For this review, take the finished solid that the model builds, in its own axes (mm). Face numbers are marked on the shaded views. Round coordinates to 2 decimals unless told otherwise and drop trailing zeros. Loops run counter-clockwise (first coordinate to the right, second up) from the corner with the lowest first, then second, coordinate; pieces in that order, holes last. Notation, with made-up numbers: (-0.5, 26.5) -> (14.5, 26.5) arc R29 cw to (14.5, 50.5) -> close; hole circle Ø2 at (82, 39.25). An arc over 180 degrees is marked (long way). Use one line per item in the form item = value. Start each with the question number.
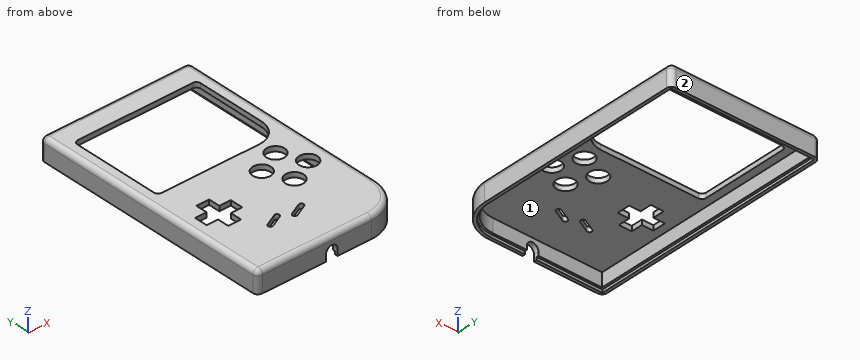
from build123d import *

# Parameters (mm, degrees)
SKETCH1_W               = 90
SKETCH1_H               = 147.5
BOSS_EXTRUDE1_DEPTH     = 13
ROUNDED_BOTTOM_CORNER_R = 21
ROUND_EDGES_R           = 3
SHELL2_DEPTH            = 10
CUT_EXTRUDE1_DEPTH      = 88.367399526
CUT_EXTRUDE2_DEPTH      = 1.75
CUT_EXTRUDE3_REACH      = 156.759
SKETCH6_R               = 5.5
CUT_EXTRUDE4_DEPTH      = 88.367399526
SKETCH7_W               = 7.75
SKETCH7_H               = 21.6
SKETCH7_W_2             = 21.6
SKETCH7_H_2             = 7.75
CUT_EXTRUDE5_DEPTH      = 88.367399526
CUT_EXTRUDE6_DEPTH      = 88.367399526


# Read off the part's stored shape, not the designer's step: Shell2
with BuildPart() as part:
    # Sketch1 → Boss-Extrude1 (new body)
    with BuildSketch(Plane.XY):
        Rectangle(SKETCH1_W, SKETCH1_H)
    extrude(amount=BOSS_EXTRUDE1_DEPTH)

    # Rounded Bottom Corner
    rounded_bottom_corner_edges = [part.edges().sort_by_distance(p)[0] for p in [
        (45, -73.75, 6.5),
    ]]
    fillet(rounded_bottom_corner_edges, radius=ROUNDED_BOTTOM_CORNER_R)

    # Round Edges
    round_edges_edges = [part.edges().sort_by_distance(p)[0] for p in [
        (-45, 0, 13),
        (-10.5, -73.75, 13),
        (45, 10.5, 13),
        (38.849242405, -67.599242405, 13),
        (0, 73.75, 13),
        (-45, -73.75, 6.5),
        (-45, 73.75, 6.5),
        (45, 73.75, 6.5),
    ]]
    fillet(round_edges_edges, radius=ROUND_EDGES_R)

    # Shell2 outline → Shell2 (cut)
    with BuildSketch(Plane.XY):
        with BuildLine():
            Line((42, -52.75), (42, 70.75))
            Line((42, 70.75), (-42, 70.75))
            Line((-42, 70.75), (-42, -70.75))
            Line((-42, -70.75), (24, -70.75))
            ThreePointArc((24, -70.75), (36.727922061, -65.477922061), (42, -52.75))
        make_face()
    extrude(amount=SHELL2_DEPTH, mode=Mode.SUBTRACT)

    # Sketch2 → Cut-Extrude1 (cut, through all)
    with BuildSketch(Plane.XY.offset(13)):
        with BuildLine():
            Line((-34.75, 59.75), (34.75, 59.75))
            ThreePointArc((34.75, 59.75), (36.517766953, 59.017766953), (37.25, 57.25))
            Line((37.25, 57.25), (37.25, 15.75))
            ThreePointArc((37.25, 15.75), (33.442388155, 6.557611845), (24.25, 2.75))
            Line((24.25, 2.75), (-34.75, 2.75))
            ThreePointArc((-34.75, 2.75), (-36.517766953, 3.482233047), (-37.25, 5.25))
            Line((-37.25, 5.25), (-37.25, 57.25))
            ThreePointArc((-37.25, 57.25), (-36.517766953, 59.017766953), (-34.75, 59.75))
        make_face()
    extrude(amount=-CUT_EXTRUDE1_DEPTH, mode=Mode.SUBTRACT)

    # Sketch3 → Cut-Extrude2 (cut)
    with BuildSketch(Plane(origin=(0, 0, 0), x_dir=(-1, 0, 0), z_dir=(0, 0, -1))):
        with BuildLine():
            Line((-43.25, -52.75), (-43.25, 72))
            Line((-43.25, 72), (43.25, 72))
            Line((43.25, 72), (43.25, -72))
            Line((43.25, -72), (-24, -72))
            ThreePointArc((-24, -72), (-37.611805538, -66.361805538), (-43.25, -52.75))
        make_face()
        with BuildLine():
            Line((-42, -52.75), (-42, 70.75))
            Line((-42, 70.75), (42, 70.75))
            Line((42, 70.75), (42, -70.75))
            Line((42, -70.75), (-24, -70.75))
            ThreePointArc((-24, -70.75), (-36.727922061, -65.477922061), (-42, -52.75))
        make_face(mode=Mode.SUBTRACT)
    extrude(amount=-CUT_EXTRUDE2_DEPTH, mode=Mode.SUBTRACT)

    # Sketch4 → Cut-Extrude3 (cut, up to next)
    with BuildSketch(Plane.XZ.offset(73.75), mode=Mode.PRIVATE) as cut_extrude3_sk1:
        with BuildLine():
            Line((-3.5, 0), (3.5, 0))
            Line((3.5, 0), (3.5, 4))
            ThreePointArc((3.5, 4), (0, 7.5), (-3.5, 4))
            Line((-3.5, 4), (-3.5, 0))
        make_face()
    cut_extrude3_tool1 = extrude(cut_extrude3_sk1.sketch, amount=-CUT_EXTRUDE3_REACH, mode=Mode.PRIVATE) & part.part
    add(cut_extrude3_tool1.solids().sort_by_distance((0, -73.75, 3.419658))[0], mode=Mode.SUBTRACT)

    # Sketch6 → Cut-Extrude4 (cut, through all)
    with BuildSketch(Plane.XY.offset(13)):
        with Locations((32, -21.75)):
            Circle(SKETCH6_R)
        with Locations((17.546893068, -28.66)):
            Circle(SKETCH6_R)
        with Locations((25.098626717, -7.314936896)):
            Circle(SKETCH6_R)
        with Locations((10.645519784, -14.224936896)):
            Circle(SKETCH6_R)
    extrude(amount=-CUT_EXTRUDE4_DEPTH, mode=Mode.SUBTRACT)

    # Sketch7 → Cut-Extrude5 (cut, through all)
    with BuildSketch(Plane.XY.offset(13)):
        with Locations((-26.15, -26.31)):
            Rectangle(SKETCH7_W, SKETCH7_H)
        with Locations((-26.15, -26.31)):
            Rectangle(SKETCH7_W_2, SKETCH7_H_2)
    extrude(amount=-CUT_EXTRUDE5_DEPTH, mode=Mode.SUBTRACT)

    # Sketch8 → Cut-Extrude6 (cut, through all)
    with BuildSketch(Plane.XY.offset(13)):
        with BuildLine():
            Line((-2.01359375, -48.949501032), (5.145672972, -45.379501032))
            ThreePointArc((5.145672972, -45.379501032), (6.98976569, -45.99640625), (6.372860472, -47.840498968))
            Line((6.372860472, -47.840498968), (-0.78640625, -51.410498968))
            ThreePointArc((-0.78640625, -51.410498968), (-2.630498968, -50.79359375), (-2.01359375, -48.949501032))
        make_face()
        with BuildLine():
            Line((-15.98359375, -48.099501032), (-8.824327028, -44.529501032))
            ThreePointArc((-8.824327028, -44.529501032), (-6.98023431, -45.14640625), (-7.597139528, -46.990498968))
            Line((-7.597139528, -46.990498968), (-14.75640625, -50.560498968))
            ThreePointArc((-14.75640625, -50.560498968), (-16.600498968, -49.94359375), (-15.98359375, -48.099501032))
        make_face()
    extrude(amount=-CUT_EXTRUDE6_DEPTH, mode=Mode.SUBTRACT)


solid = part.part
Item 1: Wall thickness on line 1 (X direction, y = -3, z = 5.75); line 2 (Y direction, x = 10, z = 5.25); line 3 (Y direction, x = -14, z = 10.5): over which ranges is each line inside the solid? List them lowest first.
Item 2: Take a section at B-B on y = 37.5. Give the boundary of the cut face in (x, z).
Item 3: Take a section at A-A on x = -19.5. Give the boundary of the cut face in (y, z) (3 decimals).
Item 4: Take a section at D-D on x = 29. Give the number of separate pieces and of enclosed holes in the cut face, plus the area to 3 significant figures.
Item 5: For P1, Ø12, axis at x = -10, y = -1, coming from the -Z side; P2, Ø2.5, axis at y = -28, z = 12, coming from the +X side; P3, Ø0.9, axis at x = -34.5, z = 12, coming from the -Y side; P4, Ø10, axis at x = 32, y = -21.75, coming from the +Z side, all flat-tipped, find the tip position at first contact; note any pin that passes through.
Item 6: Take a section at C-C on y = -28.66. Give the boundary of the cut face in (x, z), plus the area to 3 significant figures.
Item 7: Draft analysis for pull direction X (two halves, no side actions). For the marked faces 1 and 2, state which applies: +X half, -X half, draft (parallel to the pull), parting line (faces both ways), or undercut.
Results:
q1.line_1 = -45 to -42, 42 to 45
q1.line_2 = -73.75 to -70.75, 70.75 to 73.75
q1.line_3 = -73.71 to -50.18, -47.11 to 2.75, 59.75 to 73.71
q2.outline = (-45, 0) -> (-43.25, 0) -> (-43.25, 1.75) -> (-42, 1.75) -> (-42, 10) -> (-37.25, 10) -> (-37.25, 13) -> (-42, 13) arc R3 ccw to (-45, 10) -> close; (37.25, 10) -> (42, 10) -> (42, 1.75) -> (43.25, 1.75) -> (43.25, 0) -> (45, 0) -> (45, 10) arc R3 ccw to (42, 13) -> (37.25, 13) -> close
q3.outline = (-73.75, 0) -> (-72, 0) -> (-72, 1.75) -> (-70.75, 1.75) -> (-70.75, 10) -> (-30.185, 10) -> (-30.185, 13) -> (-70.75, 13) arc R3 ccw to (-73.75, 10) -> close; (-22.435, 10) -> (2.75, 10) -> (2.75, 13) -> (-22.435, 13) -> close; (59.75, 10) -> (70.75, 10) -> (70.75, 1.75) -> (72, 1.75) -> (72, 0) -> (73.75, 0) -> (73.75, 10) arc R3 ccw to (70.75, 13) -> (59.75, 13) -> close
q4.separate_pieces = 4
q4.enclosed_holes = 0
q4.area = 274 mm2
q5.P1 = 10
q5.P2 = 44.9
q5.P3 = -73.32
q5.P4 = through
q6.outline = (-45, 0) -> (-43.25, 0) -> (-43.25, 1.75) -> (-42, 1.75) -> (-42, 10) -> (-36.95, 10) -> (-36.95, 13) -> (-42, 13) arc R3 ccw to (-45, 10) -> close; (-15.35, 10) -> (12.05, 10) -> (12.05, 13) -> (-15.35, 13) -> close; (23.05, 10) -> (42, 10) -> (42, 1.75) -> (43.25, 1.75) -> (43.25, 0) -> (45, 0) -> (45, 10) arc R3 ccw to (42, 13) -> (23.05, 13) -> close
q6.area = 224 mm2
q7.face_1 = undercut
q7.face_2 = draft
